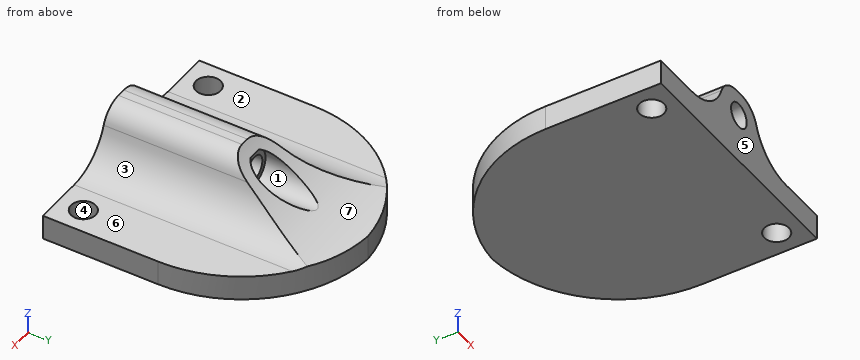
```python
from build123d import *

# Parameters (mm, degrees)
F0_W        = 50
F0_H        = 50
F0_R        = 2.5
F1_DEPTH    = 5
F2_R        = 2.5
F3_DEPTH    = 50
F4_R        = 5
F6_DEPTH    = 50
F7_R        = 3.5
F8_DEPTH    = 23
F9_T1_DEPTH = 138.5987158


# Not quite as in the source:
# - a fillet or chamfer that OpenCascade refuses, or shapes differently, is made with other operations: its cross-section is extruded or revolved along the edge and cut away or added


with BuildPart() as f1:
    # F0 (on Top) → F1 (new body)
    with BuildSketch(Plane.XY):
        Rectangle(F0_W, F0_H)
        with Locations((-20, -20)):
            Circle(F0_R, mode=Mode.SUBTRACT)
        with Locations((20, -20)):
            Circle(F0_R, mode=Mode.SUBTRACT)
    extrude(amount=F1_DEPTH)

    # F2 (on face) → F3 (join, through all)
    with BuildSketch(Plane.XZ.offset(25)):
        with BuildLine():
            Line((-5, 5), (5, 5))
            Line((5, 5), (15, 5))
            ThreePointArc((15, 5), (7.9289321881, 7.9289321881), (5, 15))
            Line((5, 15), (-5, 15))
            ThreePointArc((-5, 15), (-7.9289321881, 7.9289321881), (-15, 5))
            Line((-15, 5), (-5, 5))
        make_face()
        with Locations((0, 10)):
            Circle(F2_R, mode=Mode.SUBTRACT)
    extrude(amount=-F3_DEPTH)

    # F4
    f4_edges = [f1.edges().sort_by_distance(p)[0] for p in [
        (-5, 0, 15),
        (5, 0, 15),
    ]]
    fillet(f4_edges, radius=F4_R)

    # F5 (on face) → F6 (cut, through all)
    with BuildSketch(Plane(origin=(-25, 0, 0), x_dir=(0, -1, 0), z_dir=(-1, 0, 0))):
        with BuildLine():
            Line((-25, 15), (-25, 5))
            ThreePointArc((-25, 5), (-11.5370879822, 7.5927199554), (0, 15))
            Line((0, 15), (-25, 15))
        make_face()
    extrude(amount=-F6_DEPTH, mode=Mode.SUBTRACT)

    # F7 (on face) → F8 (cut)
    with BuildSketch(Plane(origin=(0, 25, 0), x_dir=(-1, 0, 0), z_dir=(0, 1, 0))):
        with Locations((0, 10)):
            Circle(F7_R)
    extrude(amount=-F8_DEPTH, mode=Mode.SUBTRACT)

    # F9: fillet of radius 26.71974316 on 2 edges, made by hand

    # F9_s2 → F9_t1 (cut)
    with BuildSketch(Plane.XY.offset(-66.7993579)):
        with BuildLine():
            ThreePointArc((-1.71974316, 25), (17.17396842, 17.17396842), (25, -1.71974316))
            Line((25, -1.71974316), (25, 25))
            Line((25, 25), (-1.71974316, 25))
        make_face()
        with BuildLine():
            ThreePointArc((1.71974316, 25), (-17.17396842, 17.17396842), (-25, -1.71974316))
            Line((-25, -1.71974316), (-25, 25))
            Line((-25, 25), (1.71974316, 25))
        make_face()
    extrude(amount=F9_T1_DEPTH, mode=Mode.SUBTRACT)


solid = f1.part
```
Check sheet for the modelled part. Datum: model origin and axes. Units: mm. Face numbers are marked on the shaded views. A direction names the side the tool comes from. Coordinates: 2 decimals unless noted, no trailing zeros. Write each loop counter-clockwise with the first axis right and the second up, starting at its lowest first coordinate (ties: lowest second). Pieces come first, ordered by that corner, then holes. Notation, with made-up numbers: (73.5, 64) -> (109.5, 64) arc R21 ccw to (109.5, 79) -> close; hole circle Ø2 at (-19, 30.5). An arc over 180 degrees is marked (long way). Use a Markdown table: item, result.
1. Sectioned sample at C-C (z = 10). Enter the section's corners in (x, y), plus the area to 3 significant figures.
Reported:
| item | result |
|---|---|
| outline | (-6.34, -25) -> (-2.5, -25) -> (-2.5, 2) -> (-3.5, 2) -> (-3.5, 6.63) -> (-6.34, 6.63) -> close; (2.5, -25) -> (6.34, -25) -> (6.34, 6.63) -> (3.5, 6.63) -> (3.5, 2) -> (2.5, 2) -> close |
| area | 234 mm2 |
2. Sectioned sample at D-D (y = 13.5). Enter the section's corners in (x, z), plus the area to 3 significant figures.
Reported:
| item | result |
|---|---|
| outline | (-20.24, 0) -> (20.24, 0) -> (20.24, 5) -> (15, 5) arc R10 cw to (9.17, 6.87) -> (1.57, 6.87) arc R3.5 cw to (-1.57, 6.87) -> (-9.17, 6.87) arc R10 cw to (-15, 5) -> (-20.24, 5) -> close |
| area | 243 mm2 |
3. Go/stop test with flat-tipped pins: pin 1 Ø3 at (x, y) = (20, -20) entering from +Z; pin 2 Ø5 at (x, y) = (-8.5, -15.5) entering from +Z; pin 3 Ø5 at (y, z) = (3, 1.5) entering from -X; pin 4 Ø12 at (x, y) = (-17.5, 2) entering from +Z. Record where each tip stops, or that it passes through.
Reported:
| item | result |
|---|---|
| pin 1 | passes through |
| pin 2 | stops at z = 10.64 |
| pin 3 | stops at x = -24.91 |
| pin 4 | stops at z = 5.63 |
4. Sectioned sample at A-A (y = -16). Enter the section's corners in (x, z).
Reported:
| item | result |
|---|---|
| outline | (-25, 0) -> (25, 0) -> (25, 5) -> (15, 5) arc R10 cw to (5.57, 11.67) arc R5 ccw to (0.86, 15) -> (-0.86, 15) arc R5 ccw to (-5.57, 11.67) arc R10 cw to (-15, 5) -> (-25, 5) -> close; hole circle Ø5 at (0, 10) |
5. Sectioned sample at B-B (x = 20). Enter the section's corners in (y, z), plus the area to 3 significant figures.
Reported:
| item | result |
|---|---|
| outline | (-25, 0) -> (-22.5, 0) -> (-22.5, 5) -> (-25, 5) -> close; (-17.5, 0) -> (13.84, 0) -> (13.84, 5) -> (-17.5, 5) -> close |
| area | 169 mm2 |
6. Release check for a two-part mould opening along Y. For the marked faces 4, 5, 6 and 7 record: pulls with the +Y half, pulls with the -Y half, needs draft (parallel to the pull), parting line crosses it, or undercut.
Reported:
| item | result |
|---|---|
| face 4 | undercut |
| face 5 | pulls with the -Y half |
| face 6 | needs draft |
| face 7 | pulls with the +Y half |
7. Scan lines: line 1 along Z through (x, y) = (0, 9.5); line 2 along Y through (x, z) = (20, 3.45); line 3 along Z through (x, y) = (22, -11.5). Record each from-to range of solid material in increasing order.
Reported:
| item | result |
|---|---|
| line 1 | z = 0 to 6.5 |
| line 2 | y = -25 to -22.5, -17.5 to 13.84 |
| line 3 | z = 0 to 5 |
8. Tool access check on the marked faces 1, 2 and 3. Record the directions out of +Z, -Z, +X, -X, +Y, -Y that give a thin tool (end or side, any length) a straight path to the whole face; none if there is none.
Reported:
| item | result |
|---|---|
| face 1 | +Y |
| face 2 | +Z, -X, +Y, -Y |
| face 3 | +Z, +X, +Y, -Y |
